from build123d import *

# Parameters (mm, degrees)
SKETCH1_R           = 4
BOSS_EXTRUDE1_DEPTH = 0.5


with BuildPart() as part:
    # Sketch1 → Boss-Extrude1 (new, symmetric)
    with BuildSketch(Plane(origin=(0, 0, 0), x_dir=(1, 0, 0), z_dir=(0, 1, 0))):
        with BuildLine():
            Line((25, 325.804578988), (25, 293.304578988))
            Line((25, 293.304578988), (-25, 293.304578988))
            Line((-25, 293.304578988), (-25, 325.804578988))
            ThreePointArc((-25, 325.804578988), (-26.053340487, 325.722039688), (-27.106408582, 325.636094902))
            Line((-27.106408582, 325.636094902), (-27.946991052, 335.243996502))
            Line((-27.946991052, 335.243996502), (-31.601486967, 377.015075947))
            Line((-31.601486967, 377.015075947), (-15.662371798, 378.409567831))
            Line((-15.662371798, 378.409567831), (-12, 336.548466633))
            ThreePointArc((-12, 336.548466633), (0, 336.762335175), (12, 336.548466633))
            Line((12, 336.548466633), (15.662371798, 378.409567831))
            Line((15.662371798, 378.409567831), (31.601486967, 377.015075947))
            Line((31.601486967, 377.015075947), (27.946991052, 335.243996502))
            Line((27.946991052, 335.243996502), (27.106408582, 325.636094902))
            ThreePointArc((27.106408582, 325.636094902), (26.053340487, 325.722039688), (25, 325.804578988))
        make_face()
        with Locations(Location((-21.5, 333.754934474, 0), (0, 0, 270))):
            Circle(SKETCH1_R, mode=Mode.SUBTRACT)
        with Locations(Location((21.5, 333.754934474, 0), (0, 0, 90))):
            Circle(SKETCH1_R, mode=Mode.SUBTRACT)
        with BuildLine():
            Line((-19, 320.098149951), (-19, 309.554578988))
            ThreePointArc((-19, 309.554578988), (-15, 305.554578988), (-11, 309.554578988))
            Line((-11, 309.554578988), (-11, 320.098149951))
            ThreePointArc((-11, 320.098149951), (-15, 324.098149951), (-19, 320.098149951))
        make_face(mode=Mode.SUBTRACT)
        with BuildLine():
            Line((19, 320.098149951), (19, 309.554578988))
            ThreePointArc((19, 309.554578988), (15, 305.554578988), (11, 309.554578988))
            Line((11, 309.554578988), (11, 320.098149951))
            ThreePointArc((11, 320.098149951), (15, 324.098149951), (19, 320.098149951))
        make_face(mode=Mode.SUBTRACT)
    extrude(amount=BOSS_EXTRUDE1_DEPTH, both=True)


solid = part.part
Can you work these out from the model? Positions are in its coordinate system, mm. A direction names the side the tool comes from. Coordinates: 2 decimals unless noted, no trailing zeros. Loops run counter-clockwise (first coordinate to the right, second up) from the corner with the lowest first, then second, coordinate; pieces in that order, holes last. Notation, with made-up numbers: M -37.75,-9 L 8.25,-9 A19 ccw 8.25,-2 Z; hole C 21.5,10.25 d6. An arc over 180 degrees is marked long. Return JSON: item names as keys, results as strings. Group by question number.
Item 1: On a 3-axis mill with a long thin cutter (end or side, diameter ignored), from which of +Z, -Z, +X, -X, +Y, -Y can I reach the whole of each face in a straight line? I mean faces 1 (the flat face through (0, -0.5, -336)), 2 (the flat face through (13.806, 0.007, -357.186)), 3 (the cylindrical face through (14.912, 0.007, -324.097)). Say none if no direction works.
Item 2: Imagine slicing it at A-A (y = 0). Please give me the cut outline in (x, z).
Item 3: Imagine slicing it at D-D (z = -298.5). Please give me the cut outline in (x, y).
Item 4: Imagine slicing it at C-C (z = -351). Please give me the cut outline in (x, y).
Item 5: If I drill on L1, parallel to X at y = 0.45, z = -311; L2, parallel to Z at x = -16, y = -0.4; L3, parallel to X at y = -0.2, z = -331, over which ranges is the centre line in solid material (lowest first)? Write a range as from..to.
Item 6: Imagine slicing it at B-B (x = 13). Please give me the cut outline in (y, z), and give its area (3 significant figures).
Item 7: I'm going to push flat-ended pins straight in: pin 1 Ø5 at (x, z) = (15, -310.5) entering from +Y; pin 2 Ø0.5 at (y, z) = (0, -307) entering from -X. Where does each tip first touch, or does it pass through?
Item 8: Thinking about a two-plate mould opening in Z: for faces 4 (the flat face through (-13.857, 0.007, -357.772)), 5 (the cylindrical face through (-14.912, 0.007, -324.097)), 6 (the flat face through (0, 0.5, -336)), which applies, released by +Z, released by -Z, zero draft, split by the parting line, or undercut?
Verdict:
{
 "1": {"face 1": "+Z, -Z, +X, -X, -Y", "face 2": "-Z, +Y, -Y", "face 3": "+Y, -Y"},
 "2": {"outline": "M -31.6,-377.02 L -15.66,-378.41 L -12,-336.55 A336.76 ccw 12,-336.55 L 15.66,-378.41 L 31.6,-377.02 L 27.11,-325.64 A326.76 cw 25,-325.8 L 25,-293.3 L -25,-293.3 L -25,-325.8 A326.76 cw -27.11,-325.64 Z; hole C -21.5,-333.75 d8; hole M -19,-320.1 A4 ccw -11,-320.1 L -11,-309.55 A4 ccw -19,-309.55 Z; hole M 11,-320.1 A4 ccw 19,-320.1 L 19,-309.55 A4 ccw 11,-309.55 Z; hole C 21.5,-333.75 d8"},
 "3": {"outline": "M -25,-0.5 L 25,-0.5 L 25,0.5 L -25,0.5 Z"},
 "4": {"outline": "M -29.33,-0.5 L -13.26,-0.5 L -13.26,0.5 L -29.33,0.5 Z; M 13.26,-0.5 L 29.33,-0.5 L 29.33,0.5 L 13.26,0.5 Z"},
 "5": {"L1": "x = -25..-19, -11..11, 19..25", "L2": "z = -378.38..-323.97, -305.68..-293.3", "L3": "x = -27.58..-24.4, -18.6..18.6, 24.4..27.58"},
 "6": {"outline": "M -0.5,-347.98 L 0.5,-347.98 L 0.5,-323.56 L -0.5,-323.56 Z; M -0.5,-306.09 L 0.5,-306.09 L 0.5,-293.3 L -0.5,-293.3 Z", "area": "37.2 mm^2"},
 "7": {"pin 1": "passes through", "pin 2": "stops at x = -25"},
 "8": {"face 4": "released by -Z", "face 5": "undercut", "face 6": "zero draft"}
}
